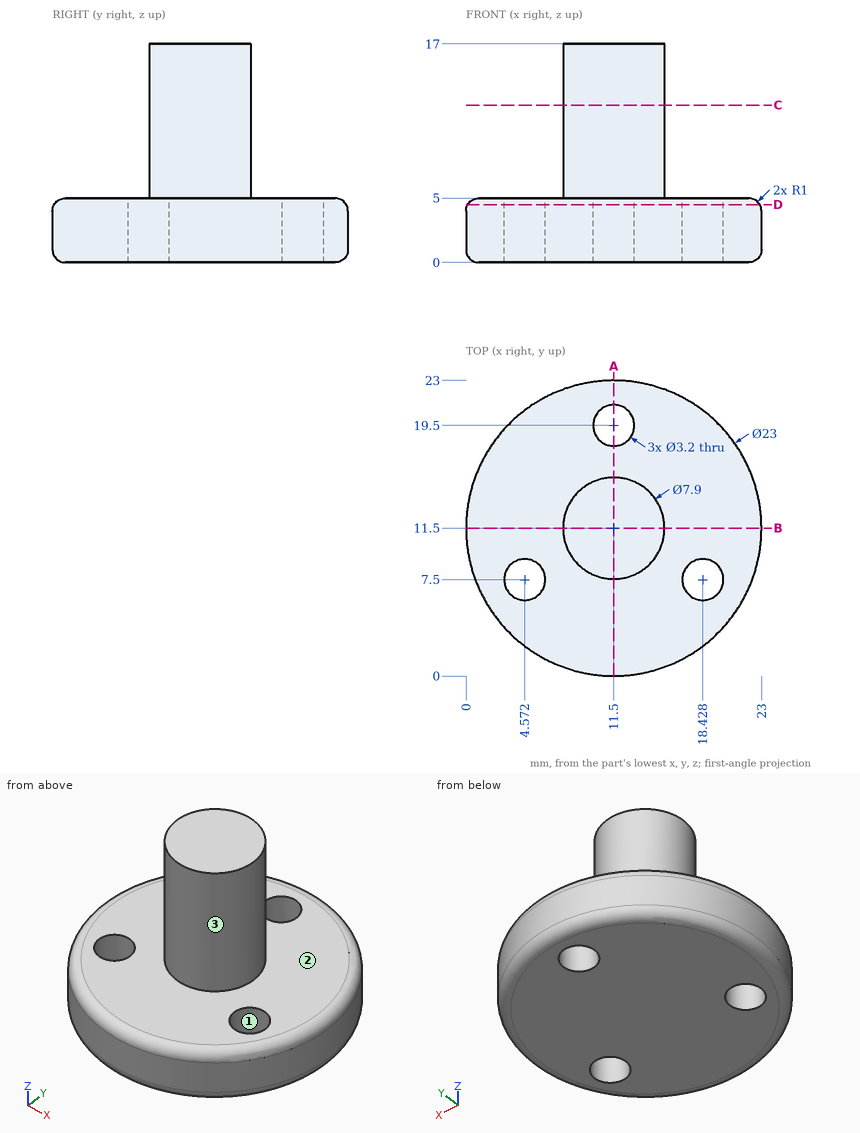
Geometry check sheet. Reference: drawing and pictorial views, mm from the part's lowest x, y, z. Coordinates: 2 decimals unless noted, no trailing zeros. Order: outer loops, then holes, each group sorted by start corner. A loop starts at its lowest first (then second) coordinate and runs counter-clockwise, first axis right, second up.
Item 1: Section check B-B, the plane y = 11.5. Enter the section's corners in (x, z).
Filled in:
outline: (0, 1) arc R1 ccw to (1, 0) - (22, 0) arc R1 ccw to (23, 1) - (23, 4) arc R1 ccw to (22, 5) - (15.45, 5) - (15.45, 17) - (7.55, 17) - (7.55, 5) - (1, 5) arc R1 ccw to (0, 4) - close
Item 2: Material ranges on L1, parallel to Y at x = 11.5, z = 2.75; L2, parallel to X at y = 7.5, z = 1.6; L3, parallel to Z at x = 20.75, y = 16.5, recorded low to high.
Filled in:
L1: y = 0 to 17.9, 21.1 to 23
L2: x = 0.72 to 2.97, 6.17 to 16.83, 20.03 to 22.28
L3: z = 0 to 5
Item 3: Section check D-D, the plane z = 4.5. Enter the section's corners in (x, y).
Filled in:
outline: circle Ø22.73 at (11.5, 11.5); hole circle Ø3.2 at (4.57, 7.5); hole circle Ø3.2 at (11.5, 19.5); hole circle Ø3.2 at (18.43, 7.5)
Item 4: Depth check by flat-ended pin: pin 1 (10 mm diameter, centred on x = 4.5, z = 9.5, fed in from -Y) (1 decimal); pin 2 (2 mm diameter, centred on x = 20, z = 3, fed in from -Y); pin 3 (2.5 mm diameter, centred on x = 18.43, y = 7.5, fed in from +Z); pin 4 (1 mm diameter, centred on x = 3, z = 4.5, fed in from -Y). Enter the tip coordinate at first touch or a pass-through.
Filled in:
pin 1: stops at y = 1.7
pin 2: stops at y = 2.78
pin 3: passes through
pin 4: stops at y = 3.34
Item 5: Release check for a two-part mould opening along Y. For the marked faces 1, 2 and 3 record: +Y half, -Y half, draft (parallel to the pull), parting line (faces both ways), or undercut.
Filled in:
face 1: undercut
face 2: draft
face 3: parting line
Item 6: Section check C-C, the plane z = 12.25. Enter the section's corners in (x, y), then the cut area to 3 significant figures.
Filled in:
outline: circle Ø7.9 at (11.5, 11.5)
area: 49.0 mm2
Item 7: Section check A-A, the plane x = 11.5. Enter the section's corners in (y, z), then the cut area to 3 significant figures.
Filled in:
outline: (0, 1) arc R1 ccw to (1, 0) - (17.9, 0) - (17.9, 5) - (15.45, 5) - (15.45, 17) - (7.55, 17) - (7.55, 5) - (1, 5) arc R1 ccw to (0, 4) - close; (21.1, 0) - (22, 0) arc R1 ccw to (23, 1) - (23, 4) arc R1 ccw to (22, 5) - (21.1, 5) - close
area: 193 mm2
